Source: CAD feature listing. Evaluate the final solid. Frame: model axes, mm. A direction names the side the tool comes from. Coordinates: 2 decimals unless noted, no trailing zeros. Loops run counter-clockwise (first coordinate to the right, second up) from the corner with the lowest first, then second, coordinate; pieces in that order, holes last. Notation, with made-up numbers: (88.5, 45) - (112.5, 45) arc R22 cw to (112.5, 84) - close; hole circle Ø1 at (68, 4.25). An arc over 180 degrees is marked (long way). Use one line per item in the form item = value. Start each with the question number.
from build123d import *

# Parameters (mm, degrees)
BASE_W              = 101.6
BASE_H              = 101.6
BOSS_EXTRUDE2_DEPTH = 6.35
SKETCH1_R           = 1.1938
SKETCH1_R_2         = 1.2446
CUT_EXTRUDE1_DEPTH  = 73.122135992
FILLET1_R           = 2.54
SKETCH2_R           = 2.794
CUT_EXTRUDE2_DEPTH  = 2.032
CUT_EXTRUDE3_DEPTH  = 73.122135992


with BuildPart() as part:
    # Base → Boss-Extrude2 (new body)
    with BuildSketch(Plane(origin=(0, 0, 0), x_dir=(1, 0, 0), z_dir=(0, 1, 0))):
        Rectangle(BASE_W, BASE_H)
    extrude(amount=BOSS_EXTRUDE2_DEPTH)

    # Sketch1 → Cut-Extrude1 (cut, through all)
    with BuildSketch(Plane(origin=(0, 6.35, 0), x_dir=(1, 0, 0), z_dir=(0, 1, 0))):
        with Locations(Location((17.6022, 24.13, 0), (0, 0, 270))):
            Circle(SKETCH1_R)
        with Locations(Location((36.195, 24.13, 0), (0, 0, 90))):
            Circle(SKETCH1_R)
        with Locations(Location((17.6022, -24.13, 0), (0, 0, 90))):
            Circle(SKETCH1_R)
        with Locations(Location((36.195, -24.13, 0), (0, 0, 270))):
            Circle(SKETCH1_R)
        with Locations(Location((-28.9814, 0, 0), (0, 0, 270))):
            Circle(SKETCH1_R_2)
        with Locations(Location((-18.8214, 0, 0), (0, 0, 270))):
            Circle(SKETCH1_R_2)
    extrude(amount=-CUT_EXTRUDE1_DEPTH, mode=Mode.SUBTRACT)

    # Fillet1
    fillet1_edges = [part.edges().sort_by_distance(p)[0] for p in [
        (50.8, 3.175, 50.8),
        (-50.8, 3.175, 50.8),
        (-50.8, 3.175, -50.8),
        (50.8, 3.175, -50.8),
    ]]
    fillet(fillet1_edges, radius=FILLET1_R)

    # Sketch2 → Cut-Extrude2 (cut)
    with BuildSketch(Plane.XZ):
        with Locations(Location((17.6022, 24.13, 0), (0, 0, 270))):
            Circle(SKETCH2_R)
        with Locations(Location((36.195, 24.13, 0), (0, 0, 270))):
            Circle(SKETCH2_R)
        with Locations(Location((36.195, -24.13, 0), (0, 0, 270))):
            Circle(SKETCH2_R)
        with Locations(Location((17.6022, -24.13, 0), (0, 0, 270))):
            Circle(SKETCH2_R)
        with Locations(Location((-18.8214, 0, 0), (0, 0, 270))):
            Circle(SKETCH2_R)
        with Locations(Location((-28.9814, 0, 0), (0, 0, 270))):
            Circle(SKETCH2_R)
    extrude(amount=-CUT_EXTRUDE2_DEPTH, mode=Mode.SUBTRACT)

    # Sketch3 → Cut-Extrude3 (cut, through all)
    with BuildSketch(Plane(origin=(0, 6.35, 0), x_dir=(1, 0, 0), z_dir=(0, 1, 0))):
        with BuildLine():
            Line((-38.1, -10.16), (4.9022, -10.16))
            ThreePointArc((4.9022, -10.16), (6.698251224, -10.903948776), (7.4422, -12.7))
            Line((7.4422, -12.7), (7.4422, -38.1))
            ThreePointArc((7.4422, -38.1), (6.698251224, -39.896051224), (4.9022, -40.64))
            Line((4.9022, -40.64), (-38.1, -40.64))
            ThreePointArc((-38.1, -40.64), (-39.896051224, -39.896051224), (-40.64, -38.1))
            Line((-40.64, -38.1), (-40.64, -12.7))
            ThreePointArc((-40.64, -12.7), (-39.896051224, -10.903948776), (-38.1, -10.16))
        make_face()
        with BuildLine():
            Line((-38.1, 40.64), (4.9022, 40.64))
            ThreePointArc((4.9022, 40.64), (6.698251224, 39.896051224), (7.4422, 38.1))
            Line((7.4422, 38.1), (7.4422, 12.7))
            ThreePointArc((7.4422, 12.7), (6.698251224, 10.903948776), (4.9022, 10.16))
            Line((4.9022, 10.16), (-38.1, 10.16))
            ThreePointArc((-38.1, 10.16), (-39.896051224, 10.903948776), (-40.64, 12.7))
            Line((-40.64, 12.7), (-40.64, 38.1))
            ThreePointArc((-40.64, 38.1), (-39.896051224, 39.896051224), (-38.1, 40.64))
        make_face()
        with BuildLine():
            Line((20.7772, 16.51), (33.02, 16.51))
            ThreePointArc((33.02, 16.51), (34.816051224, 15.766051224), (35.56, 13.97))
            Line((35.56, 13.97), (35.56, -13.97))
            ThreePointArc((35.56, -13.97), (34.816051224, -15.766051224), (33.02, -16.51))
            Line((33.02, -16.51), (20.7772, -16.51))
            ThreePointArc((20.7772, -16.51), (18.981148776, -15.766051224), (18.2372, -13.97))
            Line((18.2372, -13.97), (18.2372, 13.97))
            ThreePointArc((18.2372, 13.97), (18.981148776, 15.766051224), (20.7772, 16.51))
        make_face()
        with BuildLine():
            Line((20.7772, 43.18), (38.1, 43.18))
            ThreePointArc((38.1, 43.18), (39.896051224, 42.436051224), (40.64, 40.64))
            Line((40.64, 40.64), (40.64, 34.29))
            ThreePointArc((40.64, 34.29), (39.896051224, 32.493948776), (38.1, 31.75))
            Line((38.1, 31.75), (20.7772, 31.75))
            ThreePointArc((20.7772, 31.75), (18.981148776, 32.493948776), (18.2372, 34.29))
            Line((18.2372, 34.29), (18.2372, 40.64))
            ThreePointArc((18.2372, 40.64), (18.981148776, 42.436051224), (20.7772, 43.18))
        make_face()
        with BuildLine():
            Line((20.7772, -31.75), (38.1, -31.75))
            ThreePointArc((38.1, -31.75), (39.896051224, -32.493948776), (40.64, -34.29))
            Line((40.64, -34.29), (40.64, -40.64))
            ThreePointArc((40.64, -40.64), (39.896051224, -42.436051224), (38.1, -43.18))
            Line((38.1, -43.18), (20.7772, -43.18))
            ThreePointArc((20.7772, -43.18), (18.981148776, -42.436051224), (18.2372, -40.64))
            Line((18.2372, -40.64), (18.2372, -34.29))
            ThreePointArc((18.2372, -34.29), (18.981148776, -32.493948776), (20.7772, -31.75))
        make_face()
    extrude(amount=-CUT_EXTRUDE3_DEPTH, mode=Mode.SUBTRACT)


solid = part.part
(1) Cut plane C-C, the plane z = 24.13. Output: boundary loops of the cut face in (x, y).
(2) Material intervals for line 1 (X direction, y = 3, z = 24.13); line 2 (Z direction, x = 3, y = 2.5); line 3 (X direction, y = 3.7, z = 0), sorted ascending.
(3) Access query for faces 1 (the face through (30, 3, 43.18)), 2 (the face through (-26.21, 1, 0.36)), 3 (the face through (50.036, 3.219, -50.076)). Directions: +Z, -Z, +X, -X, +Y, -Y. A direction counts if a zero-diameter tool reaches every point of the face in a straight line with its end or side. Return the directions, or none.
(4) Contact query for a flat-ended pin moving along its axis: pin 1 (1.7 mm diameter, centred on x = 17.5, z = 24.5, fed in from -Y). Output: stop coordinate, or through.
(5) Mould query, pull axis X, two halves, no side actions, for faces 4 (the face through (-1, 0, -1)), 5 (the face through (50.8, 3, 1)), 6 (the face through (27, 3, -16.51)). Classes: +X half, -X half, draft (parallel to the pull), parting line (faces both ways), or undercut.
(6) Cut plane D-D, the plane y = 4.5. State how many separate pieces and enclosed holes the cut face has, plus the area to 3 significant figures.
(7) Cut plane B-B, the plane x = 1.5. Output: boundary loops of the cut face in (y, z).
(8) Cut plane A-A, the plane z = 0. Output: boundary loops of the cut face in (x, y), plus the area to 3 significant figures.
Recorded:
q1.outline = (-50.8, 0) - (-40.64, 0) - (-40.64, 6.35) - (-50.8, 6.35) - close; (7.44, 0) - (14.81, 0) - (14.81, 2.03) - (16.41, 2.03) - (16.41, 6.35) - (7.44, 6.35) - close; (18.8, 2.03) - (20.4, 2.03) - (20.4, 0) - (33.4, 0) - (33.4, 2.03) - (35, 2.03) - (35, 6.35) - (18.8, 6.35) - close; (37.39, 2.03) - (38.99, 2.03) - (38.99, 0) - (50.8, 0) - (50.8, 6.35) - (37.39, 6.35) - close
q2.line_1 = -50.8 to -40.64, 7.44 to 16.41, 18.8 to 35, 37.39 to 50.8
q2.line_2 = -50.8 to -40.64, -10.16 to 10.16, 40.64 to 50.8
q2.line_3 = -50.8 to -30.23, -27.74 to -20.07, -17.58 to 18.24, 35.56 to 50.8
q3.face_1 = +Y, -Y
q3.face_2 = -Y
q3.face_3 = -Z, +X, +Y, -Y
q4.pin_1 = 2.03
q5.face_4 = draft
q5.face_5 = +X half
q5.face_6 = undercut
q6.separate_pieces = 1
q6.enclosed_holes = 11
q6.area = 6,300 mm²
q7.outline = (0, -50.8) - (6.35, -50.8) - (6.35, -40.64) - (0, -40.64) - close; (0, -10.16) - (6.35, -10.16) - (6.35, 10.16) - (0, 10.16) - close; (0, 40.64) - (6.35, 40.64) - (6.35, 50.8) - (0, 50.8) - close
q8.outline = (-50.8, 0) - (-31.78, 0) - (-31.78, 2.03) - (-30.23, 2.03) - (-30.23, 6.35) - (-50.8, 6.35) - close; (-27.74, 2.03) - (-26.19, 2.03) - (-26.19, 0) - (-21.62, 0) - (-21.62, 2.03) - (-20.07, 2.03) - (-20.07, 6.35) - (-27.74, 6.35) - close; (-17.58, 2.03) - (-16.03, 2.03) - (-16.03, 0) - (18.24, 0) - (18.24, 6.35) - (-17.58, 6.35) - close; (35.56, 0) - (50.8, 0) - (50.8, 6.35) - (35.56, 6.35) - close
q8.area = 491 mm²
